For this review, use the dimensioned drawing (mm, ordinates from the lowest corner) and the shaded views. Round coordinates to 2 decimals unless told otherwise and drop trailing zeros. Write each loop counter-clockwise with the first axis right and the second up, starting at its lowest first coordinate (ties: lowest second). Pieces come first, ordered by that corner, then holes. Notation, with made-up numbers: M 88,-16 L 112,-16 A27 ccw 112,9 Z; hole C 88.5,-12 d11. An arc over 180 degrees is marked long. Use one line per item in the form item = value. Start each with the question number.
Item 1: Add section A-A (z = 532). State the section outline as (x, y) points, and give its area (3 significant figures).
Item 2: For line 1 (X direction, y = 32, z = 498); line 2 (X direction, y = 28, z = 333.5), list the stretches that pass through material, from the lowest coordinate up. Write a range as [from, to].
Item 3: For P1, Ø1.5, axis at y = 61.5, z = 241, coming from the +X side; P2, Ø1, axis at y = 18, z = 375, coming from the +X side, all flat-tipped, find the tip position at first contact; note any pin that passes through.
Item 4: Add section B-B (x = 42.5). State the section outline as (y, z) points (1 decimal), and give its area (3 significant figures).
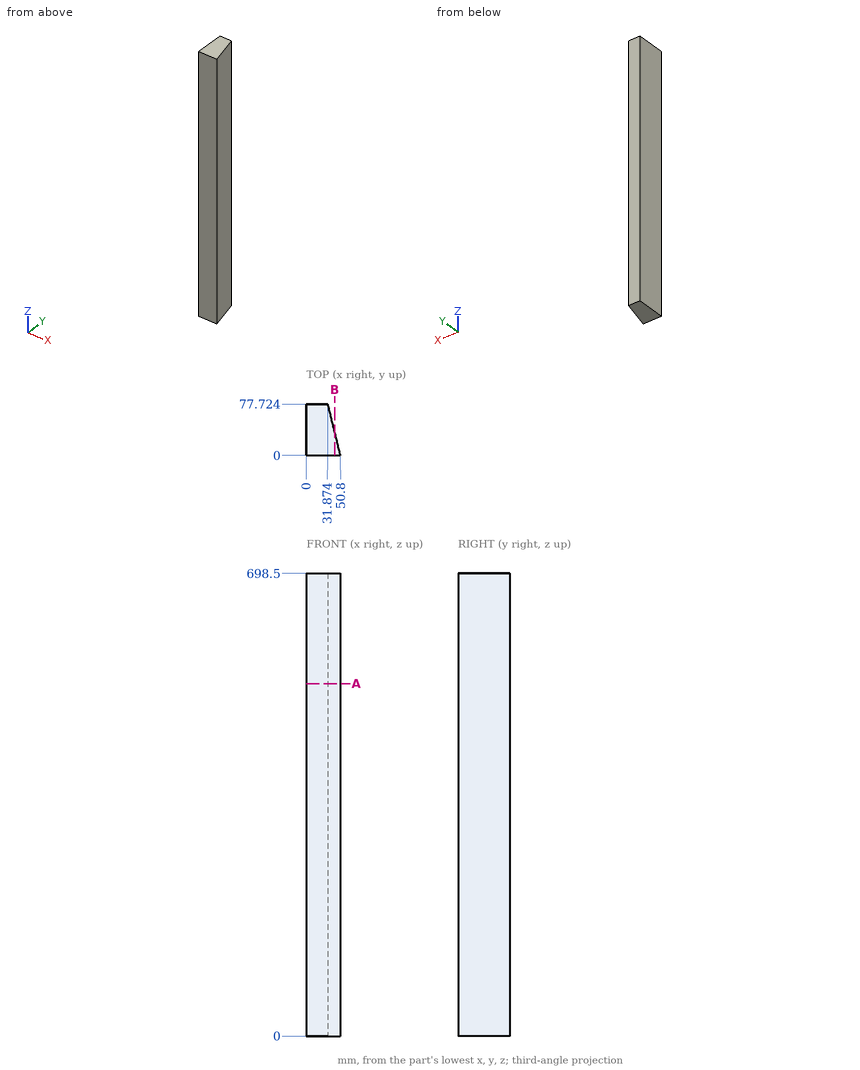
Calculated:
q1.outline = M 0,0 L 50.8,0 L 31.87,77.72 L 0,77.72 Z
q1.area = 3,210 mm^2
q2.line_1 = [0, 43.01]
q2.line_2 = [0, 43.98]
q3.P1 = 36.01
q3.P2 = 46.54
q4.outline = M 0,0 L 34.1,0 L 34.1,698.5 L 0,698.5 Z
q4.area = 23,800 mm^2
